The listing builds one solid part. Answer for the finished solid, in the listing's coordinates (mm). Coordinates: 2 decimals unless noted, no trailing zeros. Order: outer loops, then holes, each group sorted by start corner. A loop starts at its lowest first (then second) coordinate and runs counter-clockwise, first axis right, second up. Notation, with made-up numbers: (-8.75, 9) -> (42.25, 9) arc R17 cw to (42.25, 42) -> close; hole circle Ø9 at (68, 50). An arc over 180 degrees is marked (long way). Answer in a Markdown table with one row per item.
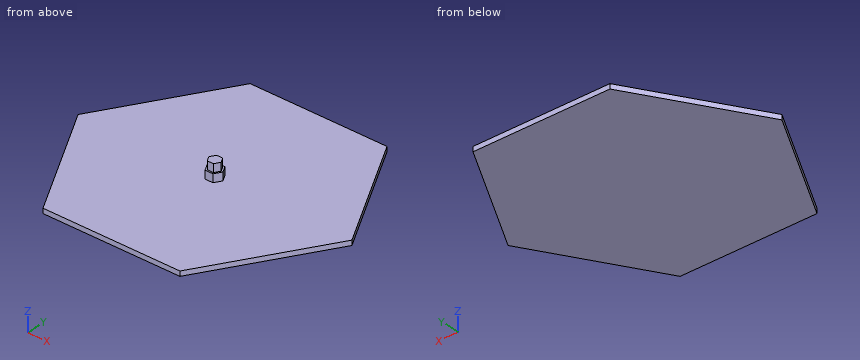
```python
from build123d import *

# Parameters (mm, degrees)
SALIENTE_EXTRUIR1_DEPTH = 3.000000026
SALIENTE_EXTRUIR2_DEPTH = 5.000000354
SALIENTE_EXTRUIR3_DEPTH = 4.999999888


with BuildPart() as part:
    # Croquis1 → Saliente-Extruir1 (new body)
    with BuildSketch(Plane(origin=(0, 0, 0), x_dir=(-1, 0, 0), z_dir=(0, 0, -1))):
        Polygon((86.602535383, 0), (43.301267691, 75), (-43.301267691, 75), (-86.602535383, 0), (-43.301267691, -75), (43.301267691, -75), align=None)
    extrude(amount=-SALIENTE_EXTRUIR1_DEPTH)

    # Croquis2 → Saliente-Extruir2 (add)
    with BuildSketch(Plane.XY.offset(3.000000026)):
        Polygon((-2.499997616, 4.330128431), (2.499997616, 4.330128431), (5.000002682, 0), (2.499997616, -4.330128431), (-2.499997616, -4.330128431), (-5.000002682, 0), align=None)
    extrude(amount=SALIENTE_EXTRUIR2_DEPTH)

    # Croquis3 → Saliente-Extruir3 (add)
    with BuildSketch(Plane.XY.offset(8.00000038)):
        Polygon((-1.949995756, -3.377497196), (-3.899998963, 0), (-1.949995756, 3.377497196), (1.949995756, 3.377497196), (3.899998963, 0), (1.949995756, -3.377497196), align=None)
    extrude(amount=SALIENTE_EXTRUIR3_DEPTH)


solid = part.part
```
(1) A cutting plane is placed at B-B, the plane x = -32. Determine the outline of the cut face in (y, z), then the cut area to 3 significant figures.
Check values:
| item | result |
|---|---|
| outline | (-75, 0) -> (75, 0) -> (75, 3) -> (-75, 3) -> close |
| area | 450 mm² |
(2) Flat-ended cylindrical pins translate along their axes: pin 1 (3 mm diameter, centred on y = 4, z = 3.5, fed in from -X); pin 2 (1.2 mm diameter, centred on x = -0.5, z = 11, fed in from +Y); pin 3 (3 mm diameter, centred on x = -49.5, y = 37.5, fed in from +Z). Find the tip coordinate at first contact, or state that the pin passes through.
Check values:
| item | result |
|---|---|
| pin 1 | x = -85.11 |
| pin 2 | y = 3.38 |
| pin 3 | z = 3 |
(3) A cutting plane is placed at C-C, the plane y = -40.5. Determine the outline of the cut face in (x, z).
Check values:
| item | result |
|---|---|
| outline | (-63.22, 0) -> (63.22, 0) -> (63.22, 3) -> (-63.22, 3) -> close |
(4) A cutting plane is placed at A-A, the plane z = 10.25. Determine the outline of the cut face in (x, y), then the cut area to 3 significant figures.
Check values:
| item | result |
|---|---|
| outline | (-3.9, 0) -> (-1.95, -3.38) -> (1.95, -3.38) -> (3.9, 0) -> (1.95, 3.38) -> (-1.95, 3.38) -> close |
| area | 39.5 mm² |
(5) Find the intervals of material crossed by line 1 along Z through (x, y) = (-41.5, -27); line 2 along X through (y, z) = (-0.5, 1); line 3 along X through (y, z) = (-2, 6.25), in increasing order. Write a range as from..to.
Check values:
| item | result |
|---|---|
| line 1 | 0..3 |
| line 2 | -86.31..86.31 |
| line 3 | -3.85..3.85 |
